Here's how the part is built. I have some questions about the finished solid (model axes, mm). Face numbers are marked on the shaded views. A direction names the side the tool comes from. Give positions to 0.01 mm unless a question says otherwise; leave off trailing zeros. Write each loop counter-clockwise with the first axis right and the second up, starting at its lowest first coordinate (ties: lowest second). Pieces come first, ordered by that corner, then holes. Notation, with made-up numbers: (-20, 66) - (-14, 66) arc R20 ccw to (-14, 93) - close; hole circle Ø2 at (81.5, -36). An arc over 180 degrees is marked (long way). Write each question's results on one line, items separated by ' | '. Start each with the question number.
Item 1: Suppose I cut it at A-A on z = 4. List the corners of the cut face in (x, y) for me, then the cut area to 3 significant figures.
Item 2: Which directions (+Z, -Z, +X, -X, +Y, -Y) give clear straight access to the entire face, cutting with the end or side of a thin tool? Please do the marked faces 1, 2 and 3.
Item 3: Suppose I cut it at D-D on y = 31.5. List the corners of the cut face in (x, z) for me, then the cut area to 3 significant figures.
Item 4: Please list where these lines run through material, in increasing order: line 1 along Z through (x, y) = (0, 48.5); line 2 along Y through (x, z) = (0, -39.75).
Item 5: Suppose I cut it at C-C on z = -17. List the corners of the cut face in (x, y) for me.
Item 6: Will these pins go through, and if not, where does the flat tip stop? P1, Ø3, axis at x = 0.5, z = 8.5, coming from the +Y side; P2, Ø2, axis at x = -2, z = -5, coming from the +Y side; P3, Ø1.5, axis at x = 0, y = -2.5, coming from the +Z side; P4, Ø3, axis at x = 0, y = -2.5, coming from the -Z side.
Item 7: Suppose I cut it at B-B on y = 45. List the corners of the cut face in (x, z) for me, then the cut area to 3 significant figures.
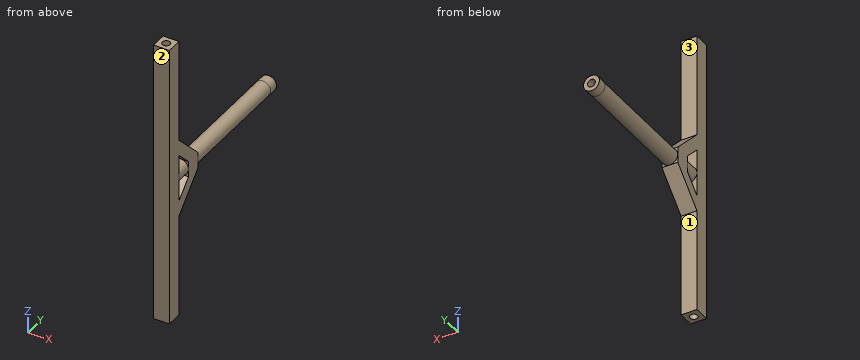
Autodesk Inventor part; units mm, degrees
ref_plane "YZ Plane" through (0, 0, 0) normal (1, 0, 0) x (0, 1, 0)
ref_plane "XZ Plane" through (0, 0, 0) normal (0, 1, 0) x (-1, 0, 0)
ref_plane "XY Plane" through (0, 0, 0) normal (0, 0, 1) x (1, 0, 0)
sketch "Szkic1" plane through (0, 0, 0) normal (0, 1, 0) x (-1, 0, 0)
  circle A0 centre (0, 0) radius 2.5
  dimension "d0" = 5
extrude "Wyciągnięcie proste1" add sketch "Szkic1" along normal blind 48
sketch "Szkic2" plane through (0, 0, 0) normal (0, -1, 0) x (1, 0, 0)
  line L0 (2.5, -45) -> (2.5, 45)
  line L1 (2.5, 45) -> (-2.5, 45)
  line L2 (-2.5, 45) -> (-2.5, -45)
  line L3 (-2.5, -45) -> (2.5, -45)
  line L4 (2.5, -45) -> (-2.5, 45) construction
  line L5 (2.5, 45) -> (-2.5, -45) construction
  point P0 (0, 0)
  dimension "d3" = 90
extrude "Wyciągnięcie proste2" add sketch "Szkic2" along normal blind 5
sketch "Szkic4" plane through (2.5, 0, -45) normal (0, 0, -1) x (-1, 0, 0)
  line L0 (5, 0) -> (5, -5)
  line L1 (5, -2.5) -> (0, -2.5)
  line L2 (0, 0) -> (0, -5)
  line L3 (0, -5) -> (5, -5)
  line L4 (2.5, -5) -> (2.5, 0)
  point P0 (2.5, -2.5)
hole "Otwór2" at (0, -2.5, -45) direction (0, 0, 1) diameter 2.459 depth 8.8 tip angle 118
sketch "Szkic5" plane through (-2.5, 0, 45) normal (0, 0, 1) x (1, 0, 0)
  line L0 (0, -5) -> (5, -5)
  line L1 (2.5, -5) -> (2.5, 0)
  line L2 (2.5, 0) -> (5, -2.5)
  line L3 (5, 0) -> (5, -5)
  line L4 (0, 0) -> (0, -5)
  line L5 (0, -2.5) -> (5, -2.5)
  circle A0 centre (2.5, -2.5) radius 1.2295
hole "Otwór3" at (0, -2.5, 45) direction (0, 0, -1) diameter 2.459 depth 8.8 tip angle 118
sketch "Szkic7" plane through (2.5, 0, 0) normal (1, 0, 0) x (0, 0, -1)
  line L0 (-45, -5) -> (45, -5)
  line L1 (-10, -5) -> (-10, 0)
  line L2 (0, -15.6) -> (0, 58.6)
  line L3 (10, -5) -> (10, 0)
  line L4 (10, -2.5) -> (-10, -2.5)
  line L5 (45, 0) -> (0, 0)
  line L6 (12.5, -5) -> (7.5, -5)
  line L7 (7.5, -5) -> (7.5, 0)
  line L8 (7.5, 0) -> (12.5, 0)
  line L9 (12.5, 0) -> (12.5, -5)
  line L10 (0, 0) -> (-45, 0)
  line L11 (-7.5, -5) -> (-12.5, -5)
  line L12 (-12.5, -5) -> (-12.5, 0)
  line L13 (-12.5, 0) -> (-7.5, 0)
  line L14 (-7.5, 0) -> (-7.5, -5)
  line L15 (2.5, 0) -> (2.5, 48)
  line L16 (2.5, 7.5) -> (-2.5498, 7.5)
  line L17 (2.5, 5) -> (-2.5, 5)
  line L18 (-2.5, 5) -> (-2.5, 10)
  line L19 (-2.5, 10) -> (2.5, 10)
  line L20 (2.5, 10) -> (2.5, 5)
  line L21 (12.5, 0) -> (2.5, 10)
  line L22 (7.5, 0) -> (2.5, 5)
  line L23 (-2.5, 5) -> (-7.5, 0)
  line L24 (-12.5, 0) -> (-2.5, 10)
  point P0 (0, -2.5)
  point P1 (0, 7.509)
  dimension "d28" = 10
  dimension "d29" = 5
  dimension "d30" = 5
  dimension "d31" = 5
  dimension "d32" = 5
extrude "Wyciągnięcie proste3" add sketch "Szkic7" against normal blind 5 contours L24 L18 L23 L10 | L19 L2 L16 L18 | L16 L2 L17 L18 | L19 L15 L16 L2 | L16 L15 L17 L2 | L21 L5 L22 L15
sketch "Szkic8" plane through (0, 48, 0) normal (0, 1, 0) x (1, 0, 0)
  circle A0 centre (0, 0) radius 2.5
extrude "Wyciągnięcie proste4" add sketch "Szkic8" along normal blind 3
sketch "Szkic9" plane through (0, 51, 0) normal (0, 1, 0) x (1, 0, 0)
  point P0 (0, 0)
  point P1 (0, 0)
hole "Otwór4" at (0, 51, 0) direction (0, -1, 0) diameter 2.459 depth 8.8 tip angle 118
properties part number "Część L1" material "Stal nierdzewna 440C"
Checked values:
1) outline: (-2.5, -5) - (2.5, -5) - (2.5, 0) - (-2.5, 0) - close; (-2.5, 3.5) - (2.5, 3.5) - (2.5, 8.5) - (-2.5, 8.5) - close | area: 50.0 mm^2
2) face 1: -Z, +X, -X, +Y | face 2: +Z, -Z, +X, -X, -Y | face 3: +Z, +X, -X, +Y
3) outline: circle Ø5 at (0, 0) | area: 19.6 mm^2
4) line 1: z = -2.5 to -1.23, 1.23 to 2.5 | line 2: y = -5 to -3.73, -1.27 to 0
5) outline: (-2.5, -5) - (2.5, -5) - (2.5, 0) - (-2.5, 0) - close
6) P1: stops at y = 5.5 | P2: stops at y = 8.5 | P3: stops at z = 35.91 | P4: stops at z = -45
7) outline: circle Ø5 at (0, 0); hole circle Ø2.46 at (0, 0) | area: 14.9 mm^2
